Read the model definition and answer for the solid it produces. Units are mm, in the model's axes. Face numbers are marked on the shaded views. Give positions to 0.01 mm unless a question says otherwise; leave off trailing zeros. Loops run counter-clockwise (first coordinate to the right, second up) from the corner with the lowest first, then second, coordinate; pieces in that order, holes last. Notation, with made-up numbers: (70, 76.25) -> (74, 76.25) arc R26 cw to (74, 110.25) -> close; hole circle Ø3 at (80.5, 89). An arc over 180 degrees is marked (long way). Write each question's results on one line, items separated by ' | '. Start each with the question number.
Item 1: Determine the mould class of the marked faces 1 and 2 for opening direction Y: +Y half, -Y half, draft (parallel to the pull), parting line (faces both ways), or undercut.
Item 2: Section B-B on z = 2.45 is taken. Write down the section's boundary in (x, y), and give its area (3 significant figures).
Item 3: Section A-A on x = 48 is taken. Write down the section's boundary in (y, z), and give its area (3 significant figures).
Item 4: Find the intervals of material crossed by line 1 (Y direction, x = 31.5, z = 1.7); line 2 (X direction, y = 9.5, z = 1.3); line 3 (Z direction, x = 29, y = 4), in increasing order.
Item 5: Section C-C on y = 14.5 is taken. Write down the section's boundary in (x, z), and give its area (3 significant figures).
```python
from build123d import *

# Parameters (mm, degrees)
F0_W     = 109
F0_H     = 55
F1_DEPTH = 1
F2_DEPTH = 3
F3_R     = 3


with BuildPart() as f1:
    # F0 (on Top) → F1 (new body)
    with BuildSketch(Plane.XY):
        with Locations((0, -3.65053)):
            Rectangle(F0_W, F0_H)
    extrude(amount=F1_DEPTH)

    # F0 (on Top) → F2 (join)
    with BuildSketch(Plane.XY):
        Polygon((56.5, 25.84947), (-56.5, 25.84947), (-56.5, -33.15053), (-11, -33.15053), (-10, -33.15053), (10, -33.15053), (11, -33.15053), (56.5, -33.15053), align=None)
        with Locations((0, -3.65053)):
            Rectangle(F0_W, F0_H, mode=Mode.SUBTRACT)
    extrude(amount=F2_DEPTH)

    # F3
    f3_edges = [f1.edges().sort_by_distance(p)[0] for p in [
        (-56.5, 25.84947, 1.5),
        (-56.5, -33.15053, 1.5),
        (56.5, -33.15053, 1.5),
        (56.5, 25.84947, 1.5),
    ]]
    fillet(f3_edges, radius=F3_R)


solid = f1.part
```
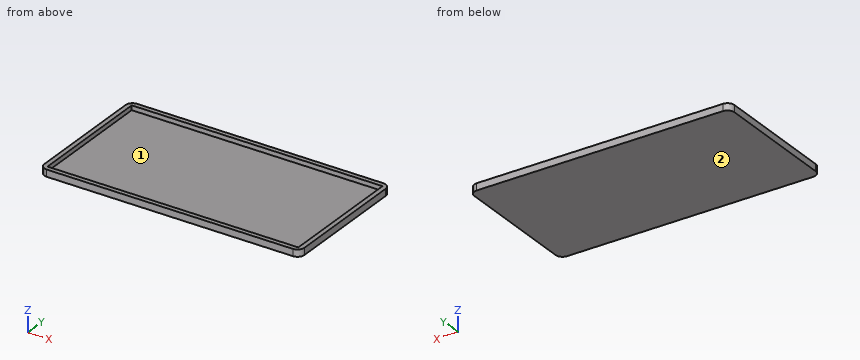
Findings:
1) face 1: undercut | face 2: draft
2) outline: (-56.5, -30.15) arc R3 ccw to (-53.5, -33.15) -> (53.5, -33.15) arc R3 ccw to (56.5, -30.15) -> (56.5, 22.85) arc R3 ccw to (53.5, 25.85) -> (-53.5, 25.85) arc R3 ccw to (-56.5, 22.85) -> close; hole (-54.5, -31.15) -> (54.5, -31.15) -> (54.5, 23.85) -> (-54.5, 23.85) -> close | area: 664 mm2
3) outline: (-33.15, 0) -> (25.85, 0) -> (25.85, 3) -> (23.85, 3) -> (23.85, 1) -> (-31.15, 1) -> (-31.15, 3) -> (-33.15, 3) -> close | area: 67.0 mm2
4) line 1: -33.15 to -31.15, 23.85 to 25.85 | line 2: -56.5 to -54.5, 54.5 to 56.5 | line 3: 0 to 1
5) outline: (-56.5, 0) -> (56.5, 0) -> (56.5, 3) -> (54.5, 3) -> (54.5, 1) -> (-54.5, 1) -> (-54.5, 3) -> (-56.5, 3) -> close | area: 121 mm2
